Can you work these out from the model? Positions are in its coordinate system, mm. A direction names the side the tool comes from. Round coordinates to 2 decimals unless told otherwise and drop trailing zeros. Order: outer loops, then holes, each group sorted by start corner. A loop starts at its lowest first (then second) coordinate and runs counter-clockwise, first axis right, second up.
Q1. For faces 1 (the face through (48, -4, 1.7)), 2 (the face through (34.217, -4.919, 10.462)), 3 (the face through (60, -4, 5)), which set-ups out of +Z, -Z, +X, -X, +Y, -Y let a thin tool reach every point of the face, with its end or its side?
Q2. If I drill on line 1 (Z direction, x = 4, y = -7.25); line 2 (Z direction, x = 8, y = -6); line 3 (Y direction, x = 40, z = 1.1), over which ranges is the centre line in solid material (lowest first)?
Q3. If we section it at C-C (z = 7): Count the separate pieces of the cut face and the enclosed holes in it, plus the area to 3 significant figures.
Q4. If we section it at A-A (z = 10.75): Please give me the cut outline in (x, y), plus the area to 3 significant figures.
Q5. We'd pull the mould along Z, two halves only. Please class faces 4 (the face through (24, -4, 1.7)), 5 (the face through (54.29, -3.94, 7.12)), 6 (the face through (-4, -4, 5)): pulls with the +Z half, pulls with the -Z half, needs draft (parallel to the pull), parting line crosses it, or undercut.
Q6. Will these pins go through, and if not, where does the flat tip stop? P1, Ø4, axis at x = 3.99, z = 6.4, coming from the +Y side; P2, Ø4.5, axis at x = 32, y = -4, coming from the -Z side.
Q7. If we section it at B-B (x = 24): Please give me the cut outline in (y, z).
from build123d import *

# Parameters (mm, degrees)
F1_DEPTH  = 8
F3_W      = 8
F3_H      = 8
F3_R      = 2.4
F4_DEPTH  = 1.7
F5_R      = 2.4
F6_DEPTH  = 1.7
F13_R     = 2.4
F14_DEPTH = 25.4


with BuildPart() as f1:
    # F0 (on Front) → F1 (new body)
    with BuildSketch(Plane.XZ):
        Polygon((-2.4, 9.6), (-4, 9.6), (-4, 0), (4, 0), (4, 9.6), (2.4, 9.6), (2.4, 11.3), (-2.4, 11.3), align=None)
    extrude(amount=F1_DEPTH)

    # F3 (on plane+point) → F4 (cut, through all)
    with BuildSketch(Plane.XY.offset(11.3)):
        with Locations((0, -4)):
            Rectangle(F3_W, F3_H)
        with Locations((0, -4)):
            Circle(F3_R, mode=Mode.SUBTRACT)
    extrude(amount=-F4_DEPTH, mode=Mode.SUBTRACT)

    # F5 (on Top) → F6 (cut)
    with BuildSketch(Plane.XY):
        with Locations((0, -4)):
            Circle(F5_R)
    extrude(amount=F6_DEPTH, mode=Mode.SUBTRACT)

    # F8: F1 across plane


with BuildPart() as f1_1:
    add(f1.part)
    add(f1.part.mirror(Plane.YZ.offset(4)))

    # F10: F1 across plane


with BuildPart() as f1_2:
    add(f1_1.part)
    add(f1_1.part.mirror(Plane.YZ.offset(12)))

    # F12: F1 across plane


with BuildPart() as f1_3:
    add(f1_2.part)
    add(f1_2.part.mirror(Plane.YZ.offset(28)))

    # F13 (on Front) → F14 (cut)
    with BuildSketch(Plane.XZ):
        with Locations((51.999, 6.4008)):
            Circle(F13_R)
        with Locations((43.998, 6.4008)):
            Circle(F13_R)
        with Locations((35.997, 6.4008)):
            Circle(F13_R)
        with Locations((27.996, 6.4008)):
            Circle(F13_R)
        with Locations((19.995, 6.4008)):
            Circle(F13_R)
        with Locations((11.994, 6.4008)):
            Circle(F13_R)
        with Locations((3.993, 6.4008)):
            Circle(F13_R)
    extrude(amount=F14_DEPTH, mode=Mode.SUBTRACT)


solid = f1_3.part
Solution:
1. face 1: -Z
1. face 2: +Z
1. face 3: +Z, -Z, +X, +Y, -Y
2. line 1: z = 0 to 4, 8.8 to 9.6
2. line 2: z = 1.7 to 11.3
2. line 3: y = -8 to -6.4, -1.6 to 0
3. separate pieces: 8
3. enclosed holes: 0
3. area: 252 mm2
4. outline: circle Ø4.8 at (0, -4); circle Ø4.8 at (8, -4); circle Ø4.8 at (16, -4); circle Ø4.8 at (24, -4); circle Ø4.8 at (32, -4); circle Ø4.8 at (40, -4); circle Ø4.8 at (48, -4); circle Ø4.8 at (56, -4)
4. area: 145 mm2
5. face 4: pulls with the -Z half
5. face 5: undercut
5. face 6: needs draft
6. P1: passes through
6. P2: stops at z = 1.7
7. outline: (-8, 0) - (-6.4, 0) - (-6.4, 1.7) - (-1.6, 1.7) - (-1.6, 0) - (0, 0) - (0, 9.6) - (-1.6, 9.6) - (-1.6, 11.3) - (-6.4, 11.3) - (-6.4, 9.6) - (-8, 9.6) - close
